from build123d import *

# Parameters (mm, degrees)
F0_R     = 11
F1_DEPTH = 7


# Not quite as in the source:
# - a feature names something its author has since deleted; it is built from what else it names


with BuildPart() as f1:
    # F0 (on Top) → F1 (new body)
    with BuildSketch(Plane.XY):
        with BuildLine():
            Line((14.175, 0), (11, 0))
            ThreePointArc((11, 0), (7.7781745931, -7.7781745931), (0, -11))
            Line((0, -11), (0, -14.175))
            ThreePointArc((0, -14.175), (4.7450574285, -13.3572098509), (8.9426071008, -10.9982))
            ThreePointArc((8.9426071008, -10.9982), (10.6919977036, -9.3065466262), (12.1262614453, -7.3406))
            ThreePointArc((12.1262614453, -7.3406), (12.4422930723, -4.2253938225), (14.0886784217, -1.561974817))
            ThreePointArc((14.0886784217, -1.561974817), (14.1534031531, -0.7821791265), (14.175, 0))
        make_face()
        with BuildLine():
            ThreePointArc((0, 11), (7.7781745931, 7.7781745931), (11, 0))
            Line((11, 0), (14.175, 0))
            ThreePointArc((14.175, 0), (10.0232386233, 10.0232386233), (0, 14.175))
            Line((0, 14.175), (0, 11))
        make_face()
        with BuildLine():
            ThreePointArc((-11, 0), (-7.7781745931, 7.7781745931), (0, 11))
            Line((0, 11), (0, 14.175))
            ThreePointArc((0, 14.175), (-4.7437129445, 13.3576873934), (-8.9403928885, 11))
            ThreePointArc((-8.9403928885, 11), (-10.6938487189, 9.304419626), (-12.1306573285, 7.3333333333))
            ThreePointArc((-12.1306573285, 7.3333333333), (-12.4461611466, 4.2234349909), (-14.0884789594, 1.5637728768))
            ThreePointArc((-14.0884789594, 1.5637728768), (-14.1533532113, 0.7830822914), (-14.175, 0))
            Line((-14.175, 0), (-11, 0))
        make_face()
        with BuildLine():
            Line((0, -14.175), (0, -11))
            ThreePointArc((0, -11), (-7.7781745931, -7.7781745931), (-11, 0))
            Line((-11, 0), (-14.175, 0))
            ThreePointArc((-14.175, 0), (-10.0232386233, -10.0232386233), (0, -14.175))
        make_face()
        with BuildLine():
            ThreePointArc((0, 14.175), (10.0232386233, 10.0232386233), (14.175, 0))
            Line((14.175, 0), (16.4338, 0))
            ThreePointArc((16.4338, 0), (19.05, 0.5089718042), (21.6662, 0))
            Line((21.6662, 0), (23.925, 0))
            ThreePointArc((23.925, 0), (32.0102886216, 12.8002359481), (47.0426071008, 10.9982))
            ThreePointArc((47.0426071008, 10.9982), (24.4514597735, 21.2483327836), (0, 17.0589086472))
            Line((0, 17.0589086472), (0, 14.175))
        make_face()
        with BuildLine():
            Line((16.4338, 0), (14.175, 0))
            ThreePointArc((14.175, 0), (14.1534031531, -0.7821791265), (14.0886784217, -1.561974817))
            ThreePointArc((14.0886784217, -1.561974817), (15.1815830564, -0.6613930561), (16.4338, 0))
        make_face()
        with BuildLine():
            ThreePointArc((-8.9403928885, 11), (-4.7437129445, 13.3576873934), (0, 14.175))
            Line((0, 14.175), (0, 17.0589086472))
            ThreePointArc((0, 17.0589086472), (-4.6644934549, 14.3161547368), (-8.9403928885, 11))
        make_face()
        with BuildLine():
            Line((0, -17.0538866478), (0, -14.175))
            ThreePointArc((0, -14.175), (-10.0232386233, -10.0232386233), (-14.175, 0))
            Line((-14.175, 0), (-16.4338, 0))
            ThreePointArc((-16.4338, 0), (-19.05, -0.5093373751), (-21.6662, 0))
            Line((-21.6662, 0), (-23.925, 0))
            ThreePointArc((-23.925, 0), (-32.0102886216, -12.8002359481), (-47.0426071008, -10.9982))
            ThreePointArc((-47.0426071008, -10.9982), (-24.4500361697, -21.2407501362), (0, -17.0538866478))
        make_face()
        with BuildLine():
            ThreePointArc((8.9426071008, -10.9982), (4.7450574285, -13.3572098509), (0, -14.175))
            Line((0, -14.175), (0, -17.0538866478))
            ThreePointArc((0, -17.0538866478), (4.6653864802, -14.3126511831), (8.9426071008, -10.9982))
        make_face()
        with BuildLine():
            ThreePointArc((12.1262614453, -7.3406), (13.4221419792, -4.55814981), (14.0886784217, -1.561974817))
            ThreePointArc((14.0886784217, -1.561974817), (12.4422930723, -4.2253938225), (12.1262614453, -7.3406))
        make_face()
        with BuildLine():
            Line((-16.4338, 0), (-14.175, 0))
            ThreePointArc((-14.175, 0), (-14.1533532113, 0.7830822914), (-14.0884789594, 1.5637728768))
            ThreePointArc((-14.0884789594, 1.5637728768), (-15.1813037797, 0.6621501584), (-16.4338, 0))
        make_face()
        with BuildLine():
            Line((23.925, 0), (21.6662, 0))
            ThreePointArc((21.6662, 0), (22.9184169436, -0.6613930561), (24.0113215783, -1.561974817))
            ThreePointArc((24.0113215783, -1.561974817), (23.9465968469, -0.7821791265), (23.925, 0))
        make_face()
        with BuildLine():
            ThreePointArc((-12.1306573285, 7.3333333333), (-13.4232162274, 4.5549853033), (-14.0884789594, 1.5637728768))
            ThreePointArc((-14.0884789594, 1.5637728768), (-12.4461611466, 4.2234349909), (-12.1306573285, 7.3333333333))
        make_face()
        with BuildLine():
            ThreePointArc((52.275, 0), (50.9002359481, 6.0897113784), (47.0426071008, 10.9982))
            ThreePointArc((47.0426071008, 10.9982), (32.0102886216, 12.8002359481), (23.925, 0))
            ThreePointArc((23.925, 0), (23.9465968469, -0.7821791265), (24.0113215783, -1.561974817))
            ThreePointArc((24.0113215783, -1.561974817), (25.6577069277, -4.2253938225), (25.9737385547, -7.3406))
            ThreePointArc((25.9737385547, -7.3406), (41.9105687904, -13.6532117281), (52.275, 0))
        make_face()
        with BuildLine():
            ThreePointArc((49.1, 0), (38.1, -11), (27.1, 0))
            ThreePointArc((27.1, 0), (38.1, 11), (49.1, 0))
        make_face(mode=Mode.SUBTRACT)
        with BuildLine():
            ThreePointArc((-25.9693426715, 7.3333333333), (-47.4033431975, 10.6947851941), (-47.0426071008, -10.9982))
            ThreePointArc((-47.0426071008, -10.9982), (-32.0102886216, -12.8002359481), (-23.925, 0))
            ThreePointArc((-23.925, 0), (-23.9466467887, 0.7830822914), (-24.0115210406, 1.5637728768))
            ThreePointArc((-24.0115210406, 1.5637728768), (-25.6538388534, 4.2234349909), (-25.9693426715, 7.3333333333))
        make_face()
        with Locations((-38.1, 0)):
            Circle(F0_R, mode=Mode.SUBTRACT)
        with BuildLine():
            ThreePointArc((25.9737385547, -7.3406), (25.6577069277, -4.2253938225), (24.0113215783, -1.561974817))
            ThreePointArc((24.0113215783, -1.561974817), (24.6778580208, -4.55814981), (25.9737385547, -7.3406))
        make_face()
        with BuildLine():
            Line((-23.925, 0), (-21.6662, 0))
            ThreePointArc((-21.6662, 0), (-22.9186962203, 0.6621501584), (-24.0115210406, 1.5637728768))
            ThreePointArc((-24.0115210406, 1.5637728768), (-23.9466467887, 0.7830822914), (-23.925, 0))
        make_face()
        with BuildLine():
            ThreePointArc((-24.0115210406, 1.5637728768), (-24.6767837726, 4.5549853033), (-25.9693426715, 7.3333333333))
            ThreePointArc((-25.9693426715, 7.3333333333), (-25.6538388534, 4.2234349909), (-24.0115210406, 1.5637728768))
        make_face()
    extrude(amount=F1_DEPTH)


solid = f1.part
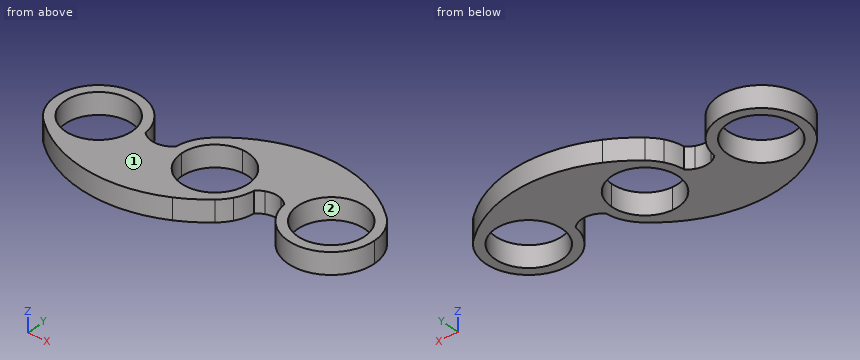
Could you check a few things on this model? Use its own coordinates, in mm. Face numbers are marked on the shaded views. Give positions to 0.01 mm unless a question says otherwise; leave off trailing zeros. Order: outer loops, then holes, each group sorted by start corner. A loop starts at its lowest first (then second) coordinate and runs counter-clockwise, first axis right, second up.
1. Suppose I cut it at B-B (z = 3.5). List the corners of the cut face in (x, y) for me (3 decimals), plus the area to 3 significant figures.
2. Suppose I cut it at A-A (x = -41.5). List the corners of the cut face in (y, z) for me.
3. Suppose I cut it at D-D (x = 38.1). List the corners of the cut face in (y, z) for me (3 decimals), plus the area to 3 significant figures.
4. Suppose I cut it at C-C (y = -4.5). List the corners of the cut face in (x, z) for me.
5. Will these pins go through, and if not, where does the flat tip stop? P1, Ø1.5, axis at y = 5.5, z = 5, coming from the -X side; P2, Ø1, axis at y = 7, z = 3.5, coming from the -X side; P3, Ø2, axis at x = 9, z = 3.5, coming from the +Y side.
6. We'd pull the mould along X, two halves only. Please class the marked faces 1 and 2: pulls with the +X half, pulls with the -X half, needs draft (parallel to the pull), parting line crosses it, or undercut.
7. I need wall thicknesses on L1, parallel to Y at x = 38.1, z = 4.25 (3 decimals); L2, parallel to Y at x = -38.1, z = 3.5 (3 decimals); L3, parallel to X at y = -5, z = 2.25. Which ranges of each line are inside material? Lowest first, please.
Solved:
1. outline: (-47.043, -10.998) arc R42.295 ccw to (8.943, -10.998) arc R14.175 ccw to (14.089, -1.562) arc R6.978 cw to (24.011, -1.562) arc R14.175 ccw (long way) to (47.043, 10.998) arc R42.271 ccw to (-8.94, 11) arc R14.175 ccw to (-14.088, 1.564) arc R6.974 cw to (-24.012, 1.564) arc R14.175 ccw (long way) to start; hole circle Ø22 at (-38.1, 0); hole circle Ø22 at (0, 0); hole circle Ø22 at (38.1, 0)
1. area: 1,700 mm2
2. outline: (-15.14, 0) - (-10.46, 0) - (-10.46, 7) - (-15.14, 7) - close; (10.46, 0) - (13.76, 0) - (13.76, 7) - (10.46, 7) - close
3. outline: (-14.175, 0) - (-11, 0) - (-11, 7) - (-14.175, 7) - close; (11, 0) - (17.059, 0) - (17.059, 7) - (11, 7) - close
3. area: 64.6 mm2
4. outline: (-51.54, 0) - (-48.14, 0) - (-48.14, 7) - (-51.54, 7) - close; (-28.06, 0) - (-10.04, 0) - (-10.04, 7) - (-28.06, 7) - close; (10.04, 0) - (13.44, 0) - (13.44, 7) - (10.04, 7) - close; (24.66, 0) - (28.06, 0) - (28.06, 7) - (24.66, 7) - close; (48.14, 0) - (51.54, 0) - (51.54, 7) - (48.14, 7) - close
5. P1: stops at x = -51.46
5. P2: stops at x = -50.7
5. P3: stops at y = 20.61
6. face 1: needs draft
6. face 2: undercut
7. L1: y = -14.175 to -11, 11 to 17.059
7. L2: y = -17.054 to -11, 11 to 14.175
7. L3: x = -51.36 to -47.9, -28.3 to -9.8, 9.8 to 13.26, 24.84 to 28.3, 47.9 to 51.36
